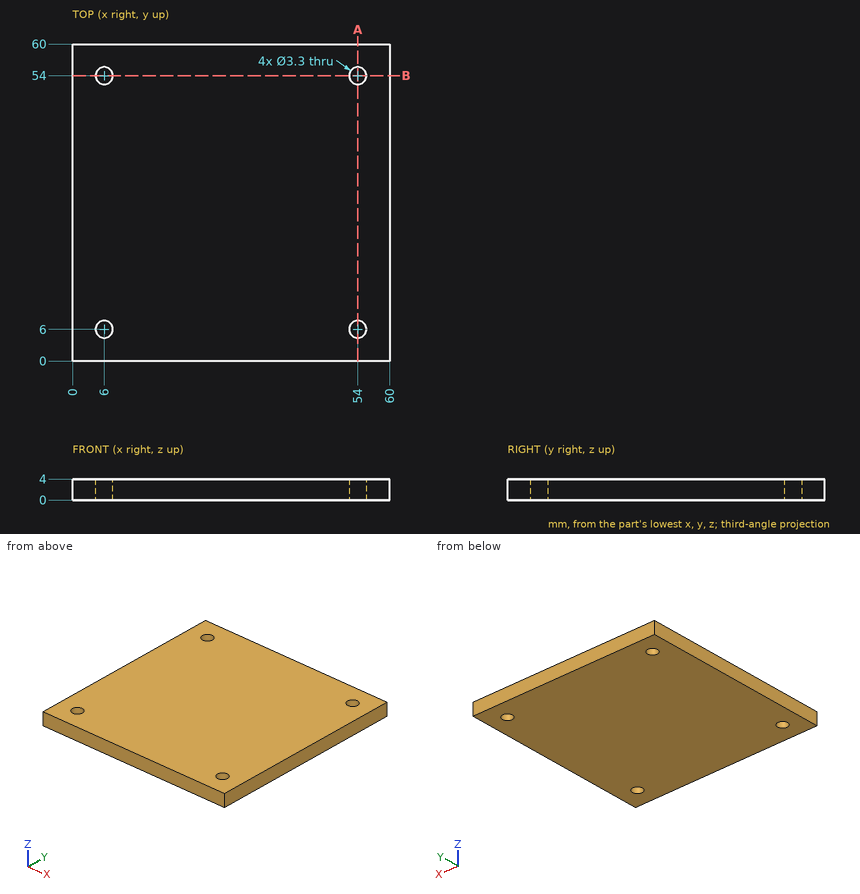
Job drawing, mm, ordinate dimensions from the low corner. One solid piece. Give positions to 0.01 mm unless a question says otherwise; leave off trailing zeros. Loops run counter-clockwise (first coordinate to the right, second up) from the corner with the lowest first, then second, coordinate; pieces in that order, holes last. Notation, with made-up numbers: M 0,80 L 51,80 A8 cw 51,95 Z; hole C 67.25,-12 d7. An arc over 180 degrees is marked long. Answer in a Markdown table with one row per item. Add a question column.
Item 1: Drop a flat-ended pin along its axis: P1, Ø8, axis at x = 13.5, y = 48, coming from the -Z side. Give the stop position or say it passes through.
Item 2: Probe probe 1 along Y at (x, z) = (54, 2.2); probe 2 along X at (y, z) = (55, 2.4); probe 3 along Y at (x, z) = (7.5, 0.95). List the from-to ranges inside material, lowest first.
Item 3: Band-saw the part on A-A on x = 54. Give the cut face in (y, z), then the cut area to 3 significant figures.
Reply:
| question | item | result |
|---|---|---|
| 1 | P1 | stops at z = 0 |
| 2 | probe 1 | y = 0 to 4.35, 7.65 to 52.35, 55.65 to 60 |
| 2 | probe 2 | x = 0 to 4.69, 7.31 to 52.69, 55.31 to 60 |
| 2 | probe 3 | y = 0 to 5.31, 6.69 to 53.31, 54.69 to 60 |
| 3 | outline | M 0,0 L 4.35,0 L 4.35,4 L 0,4 Z; M 7.65,0 L 52.35,0 L 52.35,4 L 7.65,4 Z; M 55.65,0 L 60,0 L 60,4 L 55.65,4 Z |
| 3 | area | 214 mm^2 |
